from build123d import *
from build123d.topology import SkipClean

# Parameters (mm, degrees)
BOSS_EXTRUDE1_DEPTH = 120
BOSS_EXTRUDE3_DEPTH = 7.5
BOSS_EXTRUDE2_START = 17.5
SKETCH26_R          = 19.5
SKETCH26_R_2        = 17.5
BOSS_EXTRUDE2_DEPTH = 17.5


with BuildPart() as part:
    # Sketch12 → Boss-Extrude1 (new body)
    with BuildSketch(Plane(origin=(0, 0, 0), x_dir=(1, 0, 0), z_dir=(0, 1, 0))):
        with BuildLine():
            Line((13.836638735, -11.183931196), (14.250877044, -13.310240549))
            ThreePointArc((14.250877044, -13.310240549), (19.139762737, 3.730882249), (8.20840412, 17.688191027))
            Line((8.20840412, 17.688191027), (8.634693417, 15.51841097))
            Line((8.634693417, 15.51841097), (7.567993782, 15.364331637))
            Line((7.567993782, 15.364331637), (7.375159644, 16.345842711))
            Line((7.375159644, 16.345842711), (6.621374847, 16.1773853))
            Line((6.621374847, 16.1773853), (12.217996211, -12.500838715))
            Line((12.217996211, -12.500838715), (12.971781009, -12.381940525))
            Line((12.971781009, -12.381940525), (12.790172439, -11.44177067))
            Line((12.790172439, -11.44177067), (13.836638735, -11.183931196))
        make_face()
        with BuildLine():
            ThreePointArc((15.095946542, -9.80369308), (17.668094122, 3.440704885), (10.313934488, 14.752042414))
            Line((10.313934488, 14.752042414), (10.410725736, 14.259382331))
            Line((10.410725736, 14.259382331), (8.575701021, 13.994322351))
            Line((8.575701021, 13.994322351), (13.217578727, -9.79160134))
            Line((13.217578727, -9.79160134), (15.007665389, -9.350540786))
            Line((15.007665389, -9.350540786), (15.095946542, -9.80369308))
        make_face(mode=Mode.SUBTRACT)
    extrude(amount=BOSS_EXTRUDE1_DEPTH)

    # Sketch28 → Boss-Extrude3 (add, symmetric)
    with BuildSketch(Plane.XZ):
        with BuildLine():
            Line((10.410725736, -14.259382331), (10.313927689, -14.752054328))
            ThreePointArc((10.313927689, -14.752054328), (17.668099364, -3.44070867), (15.095947667, 9.803702123))
            Line((15.095947667, 9.803702123), (15.007665389, 9.350540786))
            Line((15.007665389, 9.350540786), (13.217574825, 9.791607451))
            Line((13.217574825, 9.791607451), (8.575695107, -13.994326549))
            Line((8.575695107, -13.994326549), (10.410725736, -14.259382331))
        make_face()
    extrude(amount=BOSS_EXTRUDE3_DEPTH, both=True)

    # Sketch26 → Boss-Extrude2 (add)
    with SkipClean():  # the faces are left unmerged after this step: merging them gives an invalid solid
        with BuildSketch(Plane.XZ.offset(BOSS_EXTRUDE2_START)):
            with Locations(Location((0, 0, 0), (0, 0, 270))):
                Circle(SKETCH26_R)
            with Locations(Location((0, 0, 0), (0, 0, 45.563469932))):
                Circle(SKETCH26_R_2, mode=Mode.SUBTRACT)
        extrude(amount=-BOSS_EXTRUDE2_DEPTH)


solid = part.part
Can you work these out from the model? Positions are in its coordinate system, mm. A direction names the side the tool comes from. Round coordinates to 2 decimals unless told otherwise and drop trailing zeros. Write each loop counter-clockwise with the first axis right and the second up, starting at its lowest first coordinate (ties: lowest second). Pieces come first, ordered by that corner, then holes. Notation, with made-up numbers: M 10,-27 L 42,-27 A31 cw 42,12 Z; hole C 7.25,19 d4. An arc over 180 degrees is marked long. Use CSV: the item, a comma, the result in double quotes.
(1) I'm going to push flat-ended pins straight in: pin 1 (8 mm diameter, centred on y = 13, z = 5.5, fed in from +X); pin 2 (1 mm diameter, centred on y = 52, z = 6, fed in from +X); pin 3 (4.5 mm diameter, centred on x = 13.5, z = 1, fed in from +Y); pin 4 (6 mm diameter, centred on y = 51.5, z = 7, fed in from -X). Where does each tip first touch, or does it pass through?
Check values:
pin 1,"x = 19.44"
pin 2,"x = 18.71"
pin 3,"y = 120"
pin 4,"x = 10.56"
(2) Imagine slicing it at C-C (z = 8). Write out the boundary of the cut face in (x, y).
Check values:
outline,"M -17.78,-17.5 L -15.56,-17.5 L -15.56,0 L -17.78,0 Z; M 11.34,0 L 12.87,0 L 12.87,-7.5 L 15.56,-7.5 L 15.56,-17.5 L 17.78,-17.5 L 17.78,120 L 16.12,120 L 16.12,7.5 L 12.87,7.5 L 12.87,120 L 11.34,120 Z"
(3) Imagine slicing it at B-B (y = 102.5). Write out the boundary of the cut face in (x, z), plus the area to 3 significant figures.
Check values:
outline,"M 6.62,-16.18 L 7.38,-16.35 L 7.57,-15.36 L 8.63,-15.52 L 8.21,-17.69 A19.5 ccw 14.25,13.31 L 13.84,11.18 L 12.79,11.44 L 12.97,12.38 L 12.22,12.5 Z; hole M 8.58,-13.99 L 10.41,-14.26 L 10.31,-14.75 A18 ccw 15.1,9.8 L 15.01,9.35 L 13.22,9.79 Z"
area,"98.4 mm^2"
(4) I need wall thicknesses on line 1 along Z through (x, y) = (0, -9); line 2 along Y through (x, z) = (13, 13). Which ranges of each line are inside material? Lowest first, please.
Check values:
line 1,"-19.5 to -17.5, 17.5 to 19.5"
line 2,"-17.5 to 0"
(5) On a 3-axis mill with a long thin cutter (end or side, diameter ignored), from which of +Z, -Z, +X, -X, +Y, -Y can I reach the whole of each face in a straight line? I mean faces 4 (the flat face through (10.864, 62.962, -2.268)), 5 (the flat face through (10, 0, -2)), 6 (the flat face through (12, -17.5, 13)). Say none if no direction works.
Check values:
face 4,"+Y"
face 5,"-Y"
face 6,"+Z, -Z, +X, -X, -Y"
(6) Imagine slicing it at D-D (z = 1.5). Write out the boundary of the cut face in (x, y), plus the area to 3 significant figures.
Check values:
outline,"M -19.44,-17.5 L -17.44,-17.5 L -17.44,0 L -19.44,0 Z; M 10.07,0 L 11.6,0 L 11.6,-7.5 L 17.44,-7.5 L 17.44,-17.5 L 19.44,-17.5 L 19.44,120 L 17.94,120 L 17.94,7.5 L 11.6,7.5 L 11.6,120 L 10.07,120 Z"
area,"526 mm^2"
(7) We'd pull the mould along X, two halves only. Please class faces 1 (the flat face through (13, 7.5, -2)), 2 (the flat face through (9.38, 59.16, -2.04)), 3 (the flat face through (10.6, 120, -1.1)): +X half, -X half, draft (parallel to the pull), parting line (faces both ways), or undercut.
Check values:
face 1,"undercut"
face 2,"-X half"
face 3,"draft"
(8) Imagine slicing it at A-A (x = 0). Write out the boundary of the cut face in (y, z).
Check values:
outline,"M -17.5,-19.5 L 0,-19.5 L 0,-17.5 L -17.5,-17.5 Z; M -17.5,17.5 L 0,17.5 L 0,19.5 L -17.5,19.5 Z"
